Source: CAD feature listing. Evaluate the final solid. Frame: model axes, mm. A direction names the side the tool comes from. Give positions to 0.01 mm unless a question says otherwise; leave off trailing zeros. Loops run counter-clockwise (first coordinate to the right, second up) from the corner with the lowest first, then second, coordinate; pieces in that order, holes last. Notation, with made-up numbers: (4, 49) -> (59, 49) arc R4 ccw to (59, 54) -> close; hole circle Ø5 at (-14, 8.5). An arc over 180 degrees is marked (long way). Return JSON: item names as keys, results as strings. Group by question number.
(1) Draft query along Z for faces 4 (the face through (-21.018, 376, -2)), 5 (the face through (116, 376, -159.004)), 6 (the face through (-3, 376, -226.568)), 7 (the face through (1, 762, -18)). Return one class per face: released by +Z, released by -Z, zero draft, split by the parting line, or undercut.
(2) Ray query, line 1 (Z direction, x = -97, y = 244); line 2 (X direction, y = 514.5, z = 25.5). Return the intervals inside material, ascending. Write a range as from..to.
(3) Cut plane C-C on z = -34.5. Return loops of the section in (x, y), then the cut area to 3 significant figures.
(4) Access query for faces 1 (the face through (-209.232, 376, -193)), 2 (the face through (-116, 376, -159.004)), 3 (the face through (116, 376, 159.004)). Directions: +Z, -Z, +X, -X, +Y, -Y. A direction counts if a zero-diameter tool reaches every point of the face in a straight line with its end or side. Return the directions, or none.
(5) Cut plane A-A on x = -50. Return loops of the section in (y, z).
(6) Cut plane B-B on y = 111. Return loops of the section in (x, z).
(7) Pin query (flat end, axial travel): pin 1 (10 mm diameter, centred on y = 418.5, z = -81.5, fed in from -X). Return the tip coordinate at first contact, or that it passes through.
```python
from build123d import *

# Parameters (mm, degrees)
F1_DEPTH = 762


with BuildPart() as f1:
    # F0 (on Front) → F1 (new body)
    with BuildSketch(Plane.XZ):
        Polygon((-21.0185, 0), (0, 0), (0, 226.568), (-209.2325, 226.568), (-209.2325, 159.004), (-21.0185, 159.004), align=None)
    extrude(amount=-F1_DEPTH)

    # F2: F1 across plane


with BuildPart() as f1_1:
    add(f1.part)
    add(f1.part.mirror(Plane.XY))

    # F3: F1 across plane


with BuildPart() as f1_2:
    add(f1_1.part)
    add(f1_1.part.mirror(Plane.YZ))


solid = f1_2.part
```
Answers:
{
 "1": {"face 4": "undercut", "face 5": "undercut", "face 6": "released by -Z", "face 7": "zero draft"},
 "2": {"line 1": "-226.57..-159, 159..226.57", "line 2": "-21.02..21.02"},
 "3": {"outline": "(-21.02, 0) -> (21.02, 0) -> (21.02, 762) -> (-21.02, 762) -> close", "area": "32,000 mm²"},
 "4": {"face 1": "+Z, -Z, -X, +Y, -Y", "face 2": "-X, +Y, -Y", "face 3": "+X, +Y, -Y"},
 "5": {"outline": "(0, -226.57) -> (762, -226.57) -> (762, -159) -> (0, -159) -> close; (0, 159) -> (762, 159) -> (762, 226.57) -> (0, 226.57) -> close"},
 "6": {"outline": "(-209.23, -226.57) -> (209.23, -226.57) -> (209.23, -159) -> (21.02, -159) -> (21.02, 159) -> (209.23, 159) -> (209.23, 226.57) -> (-209.23, 226.57) -> (-209.23, 159) -> (-21.02, 159) -> (-21.02, -159) -> (-209.23, -159) -> close"},
 "7": {"pin 1": "x = -21.02"}
}
